```python
from build123d import *

# Parameters (mm, degrees)
F1_DEPTH = 75
F3_DEPTH = 25


with BuildPart() as f1:
    # F0 (on Top) → F1 (new body)
    with BuildSketch(Plane.XY):
        Polygon((0, 50), (0, 0), (42.5, 0), (42.5, 15), (70, 15), (70, 10), (95, 10), (95, -20), (115, -20), (115, 50), align=None)
    extrude(amount=F1_DEPTH)

    # F2 (on face) → F3 (cut)
    with BuildSketch(Plane.XY.offset(75)):
        Polygon((85, 50), (25, 50), (25, 0), (42.5, 0), (42.5, 15), (70, 15), (70, 10), (85, 10), align=None)
    extrude(amount=-F3_DEPTH, mode=Mode.SUBTRACT)


solid = f1.part
```
The listing builds one solid part. Answer for the finished solid, in the listing's coordinates (mm). A direction names the side the tool comes from. Round coordinates to 2 decimals unless told otherwise and drop trailing zeros. Order: outer loops, then holes, each group sorted by start corner. A loop starts at its lowest first (then second) coordinate and runs counter-clockwise, first axis right, second up. Notation, with made-up numbers: (81.5, -29.5) -> (89.5, -29.5) arc R34 cw to (89.5, 4.5) -> close; hole circle Ø4 at (67, -3.75). An arc over 180 degrees is marked (long way). Answer as CSV lines item,"result". Start each with the question number.
(1) For a pull along X with two mould halves and no side action, classify faces 5 (the face through (105, -20, 37)), 6 (the face through (55, 31, 50)), 7 (the face through (0, 25, 37)), 8 (the face through (70, 13, 25)) as +X half, -X half, draft (parallel to the pull), parting line (faces both ways), or undercut.
(2) The part is cut by section C-C (z = 33). Determine the outline of the cut face in (x, y), then the cut area to 3 significant figures.
(3) The part is cut by section A-A (z = 65). Determine the outline of the cut face in (x, y), then the cut area to 3 significant figures.
(4) Find the intervals of material crossed by probe 1 along X at (y, z) = (37, 56); probe 2 along X at (y, z) = (1, 18); probe 3 along Y at (x, z) = (92.5, 37.5), in increasing order. Write a range as from..to.
(5) A tool of negligible diameter and unlimited length cuts with its end or side. For faces 1 (the face through (57, 23, 0)), 2 (the face through (82, 10, 29)), 3 (the face through (25, 25, 63)), 4 (the face through (21, 0, 29)), from which of +Z, -Z, +X, -X, +Y, -Y can it reach the whole face along a straight path? Write none if from no direction.
(6) The part is cut by section B-B (y = 8.5). Determine the outline of the cut face in (x, z), then the cut area to 3 significant figures.
(7) The part is cut by section D-D (x = 80). Determine the outline of the cut face in (y, z).
(8) Flat-ended cylindrical pins translate along their axes: pin 1 Ø2 at (x, y) = (48, 19) entering from +Z; pin 2 Ø8 at (x, z) = (59.5, 34.5) entering from -Y; pin 3 Ø7.5 at (x, z) = (87.5, 56) entering from -Y. Find the tip coordinate at first contact, or state that the pin passes through.
Evaluation:
1,face 5,"draft"
1,face 6,"undercut"
1,face 7,"-X half"
1,face 8,"undercut"
2,outline,"(0, 0) -> (42.5, 0) -> (42.5, 15) -> (70, 15) -> (70, 10) -> (95, 10) -> (95, -20) -> (115, -20) -> (115, 50) -> (0, 50) -> close"
2,area,"5,490 mm²"
3,outline,"(0, 0) -> (25, 0) -> (25, 50) -> (0, 50) -> close; (85, 10) -> (95, 10) -> (95, -20) -> (115, -20) -> (115, 50) -> (85, 50) -> close"
3,area,"3,050 mm²"
4,probe 1,"0..25, 85..115"
4,probe 2,"0..42.5, 95..115"
4,probe 3,"10..50"
5,face 1,"-Z, +X, -X, +Y, -Y"
5,face 2,"+Z, -Z, -Y"
5,face 3,"+Z, +Y, -Y"
5,face 4,"+Z, -Z, -X, -Y"
6,outline,"(0, 0) -> (42.5, 0) -> (42.5, 50) -> (25, 50) -> (25, 75) -> (0, 75) -> close; (95, 0) -> (115, 0) -> (115, 75) -> (95, 75) -> close"
6,area,"4,250 mm²"
7,outline,"(10, 0) -> (50, 0) -> (50, 50) -> (10, 50) -> close"
8,pin 1,"z = 50"
8,pin 2,"y = 15"
8,pin 3,"y = 10"
